The drawing under review shows one solid part. Ordinate dimensions are in mm from its lowest x, y, z. A direction names the side the tool comes from. Coordinates: 2 decimals unless noted, no trailing zeros. Loops run counter-clockwise (first coordinate to the right, second up) from the corner with the lowest first, then second, coordinate; pieces in that order, holes last. Notation, with made-up numbers: (3.5, 60) - (50.5, 60) arc R16 ccw to (50.5, 80) - close; hole circle Ø11 at (-30.5, 75). An arc over 180 degrees is marked (long way). Answer as a JSON object with one key per item and string values. Group by question number.
Item 1: We need section B-B (x = 50.8). Give the boundary of the cut face in (y, z), then the cut area to 3 significant figures.
Item 2: Clearance check with a flat-ended pin moving along its axis: pin 1 (1 mm diameter, centred on x = 63, y = 40.5, fed in from +Z). State where the tip first meets the part, or that it passes through.
Item 3: To check wall thickness, follow line 1 (Y direction, x = 88, z = 18); line 2 (X direction, y = 25, z = 19); line 3 (X direction, y = 21.5, z = 47.5). State the ranges of each line that lie inside material, in increasing order.
Item 4: We need section D-D (x = 96). Give the boundary of the cut face in (y, z), then the cut area to 3 significant figures.
Item 5: Mouldability with a two-part tool opening along Y and no side actions: class the marked faces 1, 2, 3 and 4 as released by +Y, released by -Y, zero draft, split by the parting line, or undercut.
Item 6: We need section A-A (z = 10). Give the boundary of the cut face in (x, y), then the cut area to 3 significant figures.
Item 7: We need section C-C (y = 28). Give the boundary of the cut face in (x, z).
Item 8: Tool access review of the marked faces 5, 6 and 7: name each direction out of +Z, -Z, +X, -X, +Y, -Y from which nothing blocks a thin tool from reaching the whole face with its end or side.
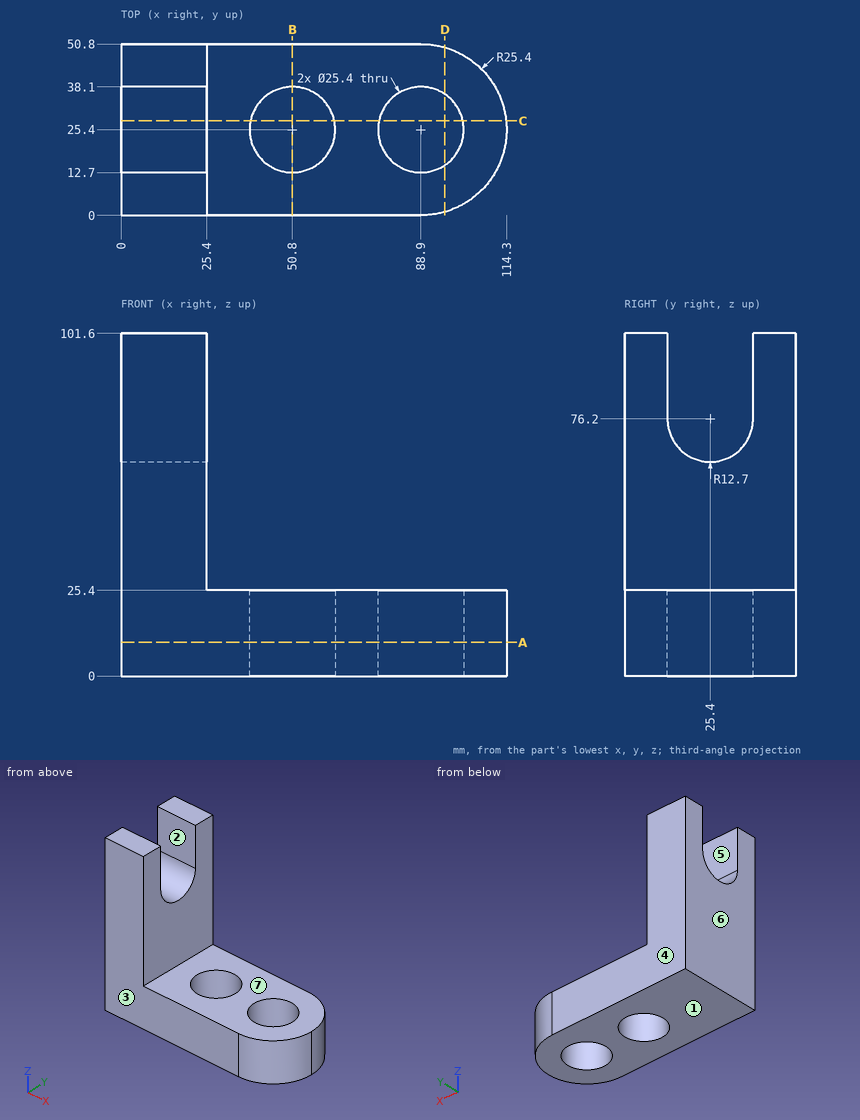
Check sheet entries:
{
 "1": {"outline": "(0, 0) - (12.7, 0) - (12.7, 25.4) - (0, 25.4) - close; (38.1, 0) - (50.8, 0) - (50.8, 25.4) - (38.1, 25.4) - close", "area": "645 mm2"},
 "2": {"pin 1": "stops at z = 25.4"},
 "3": {"line 1": "y = 0 to 12.73, 38.07 to 50.8", "line 2": "x = 0 to 38.11, 63.49 to 76.21, 101.59 to 114.3", "line 3": "x = 0 to 25.4"},
 "4": {"outline": "(1.01, 0) - (14.87, 0) - (14.87, 25.4) - (1.01, 25.4) - close; (35.93, 0) - (49.79, 0) - (49.79, 25.4) - (35.93, 25.4) - close", "area": "704 mm2"},
 "5": {"face 1": "zero draft", "face 2": "undercut", "face 3": "released by -Y", "face 4": "released by +Y"},
 "6": {"outline": "(0, 0) - (88.9, 0) arc R25.4 ccw to (88.9, 50.8) - (0, 50.8) - close; hole circle Ø25.4 at (50.8, 25.4); hole circle Ø25.4 at (88.9, 25.4)", "area": "4,520 mm2"},
 "7": {"outline": "(0, 0) - (38.37, 0) - (38.37, 25.4) - (25.4, 25.4) - (25.4, 63.77) - (0, 63.77) - close; (63.23, 0) - (76.47, 0) - (76.47, 25.4) - (63.23, 25.4) - close; (101.33, 0) - (114.17, 0) - (114.17, 25.4) - (101.33, 25.4) - close"},
 "8": {"face 5": "+Z, +X, -X", "face 6": "+Z, -Z, -X, +Y, -Y", "face 7": "+Z, +X, +Y, -Y"}
}
